```python
from build123d import *

# Parameters (mm, degrees)
F1_DEPTH = 5
F3_DEPTH = 12.5
F5_DEPTH = 1.5
F4_W     = 0.4
F4_H     = 0.65
F6_DEPTH = 15
F7_DEPTH = 7.001


with BuildPart() as f1:
    # F0 (on Front) → F1 (new body, symmetric)
    with BuildSketch(Plane.XZ):
        Polygon((-5.1, 3), (-5.1, 0), (-0.5, 0), (-0.5, -2.2), (-0.25, -3), (0.25, -3), (0.5, -2.2), (0.5, 0), (5.1, 0), (5.1, 3), (3.9, 4.2), (3.6009409723, 4.2), (2.05, 4.2), (0.4990590277, 4.2), (0.2, 4.2), (0.2, 7), (-0.2, 7), (-0.2, 4.2), (-0.4990590277, 4.2), (-2.05, 4.2), (-3.6009409723, 4.2), (-3.9, 4.2), align=None)
    extrude(amount=F1_DEPTH, both=True)

    # F2 (on Right) → F3 (intersect, symmetric)
    with BuildSketch(Plane.YZ):
        with BuildLine():
            Line((0.5, 7), (-0.5, 7))
            ThreePointArc((-0.5, 7), (-1.2071067812, 6.7071067812), (-1.5, 6))
            Line((-1.5, 6), (-1.5, 4.4))
            Line((-1.5, 4.4), (-2.9, 3))
            Line((-2.9, 3), (-2.9, -1.6))
            Line((-2.9, -1.6), (-3.4, -1.6))
            Line((-3.4, -1.6), (-3.4, -2.2))
            Line((-3.4, -2.2), (-2.6, -3))
            Line((-2.6, -3), (-2.2, -3))
            Line((-2.2, -3), (-2.2, 0))
            Line((-2.2, 0), (2.2, 0))
            Line((2.2, 0), (2.2, -3))
            Line((2.2, -3), (2.6, -3))
            Line((2.6, -3), (3.4, -2.2))
            Line((3.4, -2.2), (3.4, -1.6))
            Line((3.4, -1.6), (2.9, -1.6))
            Line((2.9, -1.6), (2.9, 3))
            Line((2.9, 3), (1.5, 4.4))
            Line((1.5, 4.4), (1.5, 6))
            ThreePointArc((1.5, 6), (1.2071067812, 6.7071067812), (0.5, 7))
        make_face()
    extrude(amount=F3_DEPTH, both=True, mode=Mode.INTERSECT)

    # F4 (on face) → F5 (join)
    with BuildSketch(Plane(origin=(0, 0, 0), x_dir=(1, 0, 0), z_dir=(0, 0, -1))):
        with BuildLine():
            ThreePointArc((-5.1, 2.45), (-4.65, 2), (-4.2, 2.45))
            ThreePointArc((-4.2, 2.45), (-4.3318019485, 2.7681980515), (-4.65, 2.9))
            ThreePointArc((-4.65, 2.9), (-4.9681980515, 2.7681980515), (-5.1, 2.45))
        make_face()
    extrude(amount=F5_DEPTH)

    # F4 (on face) → F6 (join)
    with BuildSketch(Plane(origin=(0, 0, 0), x_dir=(1, 0, 0), z_dir=(0, 0, -1))):
        with Locations((-2.75, 1.27)):
            Rectangle(F4_W, F4_H)
        with Locations((-2.75, -1.27)):
            Rectangle(F4_W, F4_H)
        with Locations((2.75, -1.27)):
            Rectangle(F4_W, F4_H)
        with Locations((2.75, 1.27)):
            Rectangle(F4_W, F4_H)
    extrude(amount=F6_DEPTH)

    # F4 (on face) → F7 (cut, through all)
    with BuildSketch(Plane(origin=(0, 0, 0), x_dir=(1, 0, 0), z_dir=(0, 0, -1))):
        Polygon((5.1, 2.9), (3.45, 2.9), (5.1, 1.25), align=None)
        Polygon((5.1, -1.25), (3.45, -2.9), (5.1, -2.9), align=None)
    extrude(amount=-F7_DEPTH, mode=Mode.SUBTRACT)

    # F0 (on Front) → F8 (revolve)
    with BuildSketch(Plane.XZ):
        with BuildLine():
            Line((-3.3430398867, 5.1812821793), (-3.6009409723, 4.2))
            Line((-3.6009409723, 4.2), (-2.05, 4.2))
            Line((-2.05, 4.2), (-1.511025513, 6.2507321944))
            ThreePointArc((-1.511025513, 6.2507321944), (-2.6485230501, 6.0954297868), (-3.3430398867, 5.1812821793))
        make_face()
    revolve(axis=Axis((-1.025, 0, 8.1), (0.2541881195, 0, 0.9671547962)))

    # F0 (on Front) → F9 (revolve)
    with BuildSketch(Plane.XZ):
        with BuildLine():
            Line((2.05, 4.2), (3.6009409723, 4.2))
            Line((3.6009409723, 4.2), (3.3430398867, 5.1812821793))
            ThreePointArc((3.3430398867, 5.1812821793), (2.6485230501, 6.0954297868), (1.511025513, 6.2507321944))
            Line((1.511025513, 6.2507321944), (2.05, 4.2))
        make_face()
    revolve(axis=Axis((1.7805127565, 0, 5.2253660972), (0.2541881195, 0, -0.9671547962)))


solid = f1.part
```
Model file for the job. Use its own axes, mm. A direction names the side the tool comes from. Coordinates: 2 decimals unless noted, no trailing zeros. Loops run counter-clockwise (first coordinate to the right, second up) from the corner with the lowest first, then second, coordinate; pieces in that order, holes last. Notation, with made-up numbers: (61, 49.25) - (83, 49.25) arc R14 ccw to (83, 69.25) - close; hole circle Ø9 at (-28, 66.5). An arc over 180 degrees is marked (long way). Write item = value, one per line. Start each with the question number.
Item 1: Wall check: probe 1 along Y at (x, z) = (-2.75, -9.75) (3 decimals); probe 2 along X at (y, z) = (1.25, -9); probe 3 along Y at (x, z) = (-3, 2.25). Give the ranges that are in metal, low to high. Write a range as [from, to].
Item 2: Saw through at A-A, the plane z = 1.5. List the corners of the cut face in (x, y), then the cut area to 3 significant figures.
Item 3: 3-axis set-ups, long thin cutter, end or side, ignore diameter. For faces 5 (the face through (0, 2.2, -1)), 6 (the face through (-1, 2.9, 1)), 7 (the face through (0.5, 2.7, -1.4)), 8 (the face through (5.1, 0, 1)): which of +Z, -Z, +X, -X, +Y, -Y reach the whole face in a straight line?
Item 4: Pull direction Y, two halves, no side cores. Call faces 1 (the face through (-0.3, 2.4, 3.5)), 2 (the face through (0, -2.2, -2)), 3 (the face through (0.2, 0, 6)), 4 (the face through (-1, -2.9, 1)): +Y half, -Y half, draft (parallel to the pull), parting line (faces both ways), or undercut.
Item 5: Drop flat-ended pins along their axis: pin 1 Ø5 at (x, z) = (-3.5, 1) entering from +Y; pin 2 Ø5 at (x, z) = (1, -9.5) entering from -Y (3 decimals); pin 3 Ø0.5 at (x, y) = (-5, -2.5) entering from -Z. Give the stop position or say it passes through.
Answers:
q1.probe_1 = [-1.595, -0.945], [0.945, 1.595]
q1.probe_2 = [-2.95, -2.55], [2.55, 2.95]
q1.probe_3 = [-2.9, 2.9]
q2.outline = (-5.1, -2.9) - (3.45, -2.9) - (5.1, -1.25) - (5.1, 1.25) - (3.45, 2.9) - (-5.1, 2.9) - close
q2.area = 56.4 mm2
q3.face_5 = -Z, +X, -X
q3.face_6 = +Z, +X, -X, +Y
q3.face_7 = -Z, +X, +Y, -Y
q3.face_8 = +Z, -Z, +X, +Y, -Y
q4.face_1 = +Y half
q4.face_2 = undercut
q4.face_3 = draft
q4.face_4 = -Y half
q5.pin_1 = 2.9
q5.pin_2 = -1.595
q5.pin_3 = -1.5
